Autodesk Inventor part; units mm, degrees
ref_plane "Flange Pattern Plane" through (12.7, 7.5406, -4.5466) normal (0, 1, 0) x (1, 0, 0)
ref_plane "YZ Plane" through (0, 0, 0) normal (1, 0, 0) x (0, 1, 0)
ref_plane "XZ Plane" through (0, 0, 0) normal (0, 1, 0) x (-1, 0, 0)
sketch "Sketch1" plane through (0, 0, 0) normal (0, 1, 0) x (-1, 0, 0)
  line L0 (-12.7, 0) -> (12.7, 0)
  line L1 (12.7, 0) -> (12.7, -12.7)
  line L2 (12.7, -12.7) -> (-12.7, -12.7)
  line L3 (-12.7, -12.7) -> (-12.7, 0)
  line L4 (12.7, 0) -> (-12.7, -12.7) construction
  point P0 (0, 0)
  point P1 (0, 0)
  dimension "d0" = 25.4
  dimension "d1" = 12.7
extrude "Plate1" add sketch "Sketch1" along normal blind 1.1906
sketch "Sketch2" plane through (11.5094, 0, -12.7) normal (1, 0, 0) x (0, 1, 0)
  line L0 (0, 12.7) -> (0, 0)
  line L1 (0, 0) -> (13.8906, 0)
  line L2 (13.8906, 0) -> (13.8906, 12.7)
  line L3 (13.8906, 12.7) -> (0, 12.7)
edge flange "Flanges" height 12.7 angle 90 thickness 1.1906 bend radius 0.7937 thickness toward (1, 0, 0) relief tear relief width 1.1906 relief depth 0.5953 corner gap 1.1906 corner form 0 edges at (12.7, 1.1906, -6.35) (-12.7, 1.1906, -6.35) wall of the first edge with corners at (11.5094, 0, 0) (11.5094, 0, -12.7) (11.5094, 13.8906, -12.7) (11.5094, 13.8906, 0)
bend "Bend1"
corner "Corner1"
sketch "Sketch3" plane through (12.7, 1.9844, -12.7) normal (1, 0, 0) x (0, 0, -1)
  line L0 (-8.1534, 7.8676) -> (-4.5466, 7.8676)
  line L1 (-4.0386, 7.3596) -> (-4.0386, 3.7528)
  line L2 (-4.5466, 3.2448) -> (-8.1534, 3.2448)
  line L3 (-8.6614, 3.7528) -> (-8.6614, 7.3596)
  arc A0 (-8.1534, 7.8676) -> (-8.6614, 7.3596) centre (-8.1534, 7.3596) ccw
  arc A1 (-4.0386, 7.3596) -> (-4.5466, 7.8676) centre (-4.5466, 7.3596) ccw
  arc A2 (-4.5466, 3.2448) -> (-4.0386, 3.7528) centre (-4.5466, 3.7528) ccw
  arc A3 (-8.6614, 3.7528) -> (-8.1534, 3.2448) centre (-8.1534, 3.7528) ccw
  line L4 (-12.7, 0) -> (-12.7, 11.9063) construction
  line L5 (-12.7, 11.9063) -> (0, 11.9063) construction
  line L6 (-8.1534, 7.3596) -> (-4.5466, 3.7528) construction
  point P0 (-12.7, -1.9844)
  point P1 (-4.0386, 3.2448)
  point P2 (-8.6614, 3.2448)
  point P3 (-6.35, 5.5562)
  dimension "d16" = 4.6228
  dimension "d17" = 0.508
  dimension "d20" = 6.35
  dimension "d21" = 6.35
extrude "Flange Stamp" cut sketch "Sketch3" against normal blind 1.1906
sketch "Sketch7" plane through (12.7, 1.9844, 0) normal (1, 0, 0) x (0, 0, -1)
  arc A0 (4.5466, 7.8676) -> (4.0386, 7.3596) centre (4.5466, 7.3596) ccw construction
  arc A1 (8.1534, 3.2448) -> (8.6614, 3.7528) centre (8.1534, 3.7528) ccw construction
  circle A2 centre (6.35, 5.5563) radius 2.1844
  line L0 (4.5466, 7.3596) -> (8.1534, 3.7528) construction
  point P0 (0, -1.9844)
  dimension "d46" = 4.3688
surface extrude "Flange Circle" sketch "Sketch7" against normal up to surface (1.1906 mm away) shown yes curves A2
ref_plane "Flange Pattern Plane" through (12.7, 7.5406, -4.5466) normal (0, 1, 0) x (1, 0, 0)
sketch "Flange Pattern Sketch" plane through (12.7, 7.5406, -4.5466) normal (0, 1, 0) x (1, 0, 0)
  line L0 (0, 3.6068) -> (0, 0) construction
  line L1 (-30.5622, -4.5466) -> (5.5732, -4.5466) construction
  line L2 (0, 0) -> (-1.1906, 0) construction
  point P0 (-12.7, -4.5466)
  point P1 (0, 1.8034)
  point P2 (0, 14.5034)
  dimension "d43" = 25.4
  dimension "d40" = 12.7
feature "Flange Pattern" [suppressed]
sketch "Sketch8" plane through (0, 0, 0) normal (0, -1, 0) x (1, 0, 0)
  line L0 (10.7156, 0) -> (-10.7156, 0) construction
  line L1 (8.1534, -4.0386) -> (4.5466, -4.0386)
  line L2 (4.0386, -4.5466) -> (4.0386, -8.1534)
  line L3 (4.5466, -8.6614) -> (8.1534, -8.6614)
  line L4 (8.6614, -8.1534) -> (8.6614, -4.5466)
  arc A0 (8.6614, -4.5466) -> (8.1534, -4.0386) centre (8.1534, -4.5466) ccw
  arc A1 (8.1534, -8.6614) -> (8.6614, -8.1534) centre (8.1534, -8.1534) ccw
  arc A2 (4.0386, -8.1534) -> (4.5466, -8.6614) centre (4.5466, -8.1534) ccw
  arc A3 (4.5466, -4.0386) -> (4.0386, -4.5466) centre (4.5466, -4.5466) ccw
  line L5 (8.1534, -4.5466) -> (4.5466, -8.1534) construction
  line L6 (12.7, 0) -> (12.7, -12.7) construction
  point P0 (0, 0)
  point P1 (4.0386, -8.6614)
  point P2 (8.6614, -8.6614)
  point P3 (6.35, -6.35)
  dimension "d49" = 4.6228
  dimension "d50" = 0.508
  dimension "d51" = 6.35
  dimension "d52" = 6.35
extrude "Body Stamp" cut sketch "Sketch8" against normal blind 1.1906
sketch "Sketch9" plane through (0, 0, 0) normal (0, -1, 0) x (1, 0, 0)
  arc A0 (8.6614, -4.5466) -> (8.1534, -4.0386) centre (8.1534, -4.5466) ccw construction
  arc A1 (4.0386, -8.1534) -> (4.5466, -8.6614) centre (4.5466, -8.1534) ccw construction
  line L0 (8.1534, -4.5466) -> (4.5466, -8.1534) construction
  circle A2 centre (6.35, -6.35) radius 2.1844
  point P0 (0, 0)
  dimension "d55" = 4.3688
surface extrude "Body Circle" sketch "Sketch9" against normal up to surface (1.1906 mm away) shown yes curves A2
sketch "Body Pattern Sketch" plane through (0, 0, 0) normal (0, -1, 0) x (1, 0, 0)
  line L0 (10.7156, 0) -> (-10.7156, 0) construction
  line L1 (12.7, 0) -> (12.7, -12.7) construction
  point P0 (0, 0)
  point P1 (6.35, -6.35)
  point P2 (6.35, -19.05)
  dimension "d62" = 12.7
  dimension "d65" = 12.7
  dimension "d58" = 6.35
  dimension "d99" = 6.35
feature "Body Pattern" [suppressed]
sketch "Sketch15" plane through (0, 0, 0) normal (0, -1, 0) x (1, 0, 0)
  line L0 (10.7156, 0) -> (-10.7156, 0) construction
  line L1 (1.8034, -10.3886) -> (-1.8034, -10.3886)
  line L2 (-2.3114, -10.8966) -> (-2.3114, -14.5034)
  line L3 (-1.8034, -15.0114) -> (1.8034, -15.0114)
  line L4 (2.3114, -14.5034) -> (2.3114, -10.8966)
  arc A0 (2.3114, -10.8966) -> (1.8034, -10.3886) centre (1.8034, -10.8966) ccw
  arc A1 (1.8034, -15.0114) -> (2.3114, -14.5034) centre (1.8034, -14.5034) ccw
  arc A2 (-1.8034, -10.3886) -> (-2.3114, -10.8966) centre (-1.8034, -10.8966) ccw
  arc A3 (-2.3114, -14.5034) -> (-1.8034, -15.0114) centre (-1.8034, -14.5034) ccw
  line L5 (1.8034, -10.8966) -> (-1.8034, -14.5034) construction
  line L6 (12.7, 0) -> (12.7, -12.7) construction
  point P0 (0, 0)
  point P1 (-2.3114, -15.0114)
  point P2 (2.3114, -15.0114)
  point P3 (0, -12.7)
  dimension "d106" = 4.6228
  dimension "d107" = 0.508
  dimension "d108" = 12.7
  dimension "d109" = 12.7
extrude "Center Stamp" cut sketch "Sketch15" against normal blind 1.1906
sketch "Sketch16" plane through (0, 0, 0) normal (0, -1, 0) x (1, 0, 0)
  circle A0 centre (0, -12.7) radius 2.1844
  line L0 (10.7156, 0) -> (-10.7156, 0) construction
  line L1 (12.7, 0) -> (12.7, -12.7) construction
  point P0 (0, 0)
  dimension "d112" = 4.3688
  dimension "d118" = 12.7
  dimension "d119" = 12.7
extrude_surface "Center Circle" [suppressed]
pattern_linear "Center Pattern" [suppressed]
sketch "Arc Length" plane through (11.5094, 1.9844, 0) normal (0, 0, 1) x (1, 0, 0)
  line L0 (0, 0) -> (1.1906, 0) construction
  arc A0 (-0.7937, -0.7938) -> (0, 0) centre (-0.7938, 0) ccw construction
  line L1 (-0.7937, -1.9844) -> (-0.7937, -0.7938) construction
  arc A1 (-0.7937, -1.9844) -> (1.1906, 0) centre (-0.7937, 0) ccw construction
  point P0 (-11.5094, -1.9844)
  dimension "d85" = 3.117
  dimension "d92" = 1.2468
sketch "Sketch13" plane through (12.7, 13.8906, 0) normal (1, 0, 0) x (0, 0, -1)
  line L0 (0, 0) -> (12.7, 0) construction
  line L1 (62.4078, 0) -> (63.4238, -1.016)
  line L2 (63.4238, -1.016) -> (64.4398, 0)
  line L3 (62.4078, 0) -> (64.4398, 0)
  line L4 (12.7, -11.9063) -> (0, -11.9063) construction
  line L5 (63.4238, -10.8903) -> (61.3168, -12.9972)
  line L6 (61.3168, -12.9972) -> (63.4238, -15.1042)
  line L7 (63.4238, -15.1042) -> (65.5308, -12.9972)
  line L8 (65.5308, -12.9972) -> (63.4238, -10.8903)
  line L9 (63.4238, -10.8903) -> (63.4238, -15.1042) construction
  line L10 (63.4238, -1.016) -> (63.4238, -10.8903) construction
  line L11 (0, -11.9063) -> (12.7, -11.9063) construction
  point P0 (0, -13.8906)
  dimension "d86" = 4.2139
  dimension "d88" = 1.016
  dimension "d91" = 1.016
  dimension "d102" = 63.4238
feature "Notch" [suppressed]
mirror "Notch Mirror" [suppressed]
pattern_linear "Notch Pattern" [suppressed]
chamfer "End Chamfer" distance 1.016 angle 45 4 edges at (-12.1047, 13.8906, -12.7) (12.1047, 13.8906, -12.7) (-12.1047, 13.8906, 0) (12.1047, 13.8906, 0)
sketch "Sketch14" plane through (-12.7, 1.9844, 431.8) normal (1, 0, 0) x (0, 0, -1)
  line L0 (431.8, 11.9063) -> (444.5, 11.9063) construction
  line L1 (431.8, 0) -> (431.8, 11.9063) construction
  line L2 (431.8, -1.9844) -> (444.5, -1.9844) construction
  line L3 (431.8, 11.9063) -> (444.5, 11.9063)
  line L4 (444.5, 11.9063) -> (444.5, -1.9844)
  line L5 (444.5, -1.9844) -> (431.8, -1.9844)
  line L6 (431.8, -1.9844) -> (431.8, 11.9063)
  point P0 (62.4078, 11.9062)
  point P1 (432.816, 11.9063)
  point P2 (431.8, 10.8903)
  point P3 (382.0521, -1.9844)
  point P4 (443.484, 11.9063)
  point P5 (254.9398, 11.9062)
  point P6 (316.4078, 11.9062)
extrude "Half Cut" cut sketch "Sketch14" along normal blind 12.7
equation "\"d1\" = 1.27 * Length"
equation "\"d18\" = Thickness"
equation "\"d53\" = Thickness"
equation "\"d89\" = Thickness"
equation "\"d2\" = Thickness"
equation "\"d3\" = BendReliefWidth"
equation "\"d4\" = BendReliefDepth"
equation "\"d5\" = MinimumRemnant"
equation "\"d6\" = TransitionRadius"
equation "\"d10\" = CornerReliefSize"
equation "\"d11\" = GapSize"
equation "\"d12\" = JacobiRadiusSize"
equation "\"BendRadius\" = Thickness"
equation "\"BendReliefWidth\" = Thickness"
equation "\"BendReliefDepth\" = 0.5 * Thickness"
equation "\"CornerReliefSize\" = 4 * Thickness"
equation "\"MinimumRemnant\" = 2 * Thickness"
equation "\"TransitionRadius\" = BendRadius"
equation "\"JacobiRadiusSize\" = BendRadius"
equation "\"GapSize\" = Thickness"
properties part number "Alu C 1x2x1x35"
Verification items for the finished model (mm, model axes). A direction names the side the tool comes from. Give positions to 0.01 mm unless a question says otherwise; leave off trailing zeros. Loops run counter-clockwise (first coordinate to the right, second up) from the corner with the lowest first, then second, coordinate; pieces in that order, holes last.
1. Set-up check for faces 1 (the flat face through (11.509, 10.5, -6.4)), 2 (the flat face through (12, 5.229, -6)), 3 (the flat face through (12.7, 11, -6)), 4 (the flat face through (2.311, 1, -12)), 5 (the flat face through (8.661, 1, -6)): record each of +Z, -Z, +X, -X, +Y, -Y from which the full face is reachable in a straight line by a thin tool's end or side.
2. Go/stop test with flat-tipped pins: pin 1 Ø6 at (y, z) = (9.5, -9) entering from -X; pin 2 Ø1 at (x, y) = (1, 0.5) entering from -Z; pin 3 Ø1 at (x, z) = (12, -6.5) entering from -Y. Record where each tip stops, or that it passes through.
3. Mould release check, pull along Z, two halves, no side actions. Record for faces 6 (the flat face through (6, 1, -4.039)), 7 (the flat face through (12, 13.891, -6)), 8 (the flat face through (12, 9.852, -6)), 9 (the flat face through (12, 5, -12.7)): released by +Z, released by -Z, zero draft, split by the parting line, or undercut.
4. Thickness scan on line 1 (X direction, y = 9, z = -3.75); line 2 (Y direction, x = 2, z = -7.25); line 3 (Z direction, x = 12.25, y = 13). Record the ranges inside material, lowest first.
5. Section check C-C, the plane z = -7.5. Enter the section's corners in (x, y), then the cut area to 3 significant figures.
6. Section check B-B, the plane y = 6.5. Enter the section's corners in (x, z).
7. Section check D-D, the plane z = -1.25. Enter the section's corners in (x, y), then the cut area to 3 significant figures.
8. Section check A-A, the plane x = 7.75. Enter the section's corners in (y, z), then the cut area to 3 significant figures.
Geometry says:
1. face 1: +Z, -Z, -X, +Y
1. face 2: +X, -X
1. face 3: +Z, -Z, +X, +Y, -Y
1. face 4: -Z, -X, +Y, -Y
1. face 5: +Y, -Y
2. pin 1: stops at x = 11.51
2. pin 2: stops at z = -10.39
2. pin 3: stops at y = 0.16
3. face 6: undercut
3. face 7: zero draft
3. face 8: undercut
3. face 9: released by -Z
4. line 1: x = 11.51 to 12.7
4. line 2: y = 0 to 1.19
4. line 3: z = -12.57 to -0.13
5. outline: (0, 0) - (4.04, 0) - (4.04, 1.19) - (0, 1.19) - close; (8.66, 0) - (10.72, 0) arc R1.98 ccw to (12.7, 1.98) - (12.7, 5.23) - (11.51, 5.23) - (11.51, 1.98) arc R0.79 cw to (10.72, 1.19) - (8.66, 1.19) - close; (11.51, 9.85) - (12.7, 9.85) - (12.7, 13.89) - (11.51, 13.89) - close
5. area: 18.5 mm2
6. outline: (11.51, -12.7) - (12.7, -12.7) - (12.7, -8.66) - (11.51, -8.66) - close; (11.51, -4.04) - (12.7, -4.04) - (12.7, 0) - (11.51, 0) - close
7. outline: (0, 0) - (10.72, 0) arc R1.98 ccw to (12.7, 1.98) - (12.7, 13.89) - (11.51, 13.89) - (11.51, 1.98) arc R0.79 cw to (10.72, 1.19) - (0, 1.19) - close
7. area: 29.5 mm2
8. outline: (0, -12.7) - (1.19, -12.7) - (1.19, -8.66) - (0, -8.66) - close; (0, -4.04) - (1.19, -4.04) - (1.19, 0) - (0, 0) - close
8. area: 9.62 mm2
